Geometry check sheet. Reference: the model listing, model coordinates, mm. A direction names the side the tool comes from. Coordinates: 2 decimals unless noted, no trailing zeros. Order: outer loops, then holes, each group sorted by start corner. A loop starts at its lowest first (then second) coordinate and runs counter-clockwise, first axis right, second up. Notation, with made-up numbers: (37, -9) - (78, -9) arc R23 cw to (78, 19) - close; hole circle Ø5 at (21, 79.25). An arc over 180 degrees is marked (long way). Return JSON: item names as keys, results as strings. Group by question number.
Item 1: Section check C-C on z = -64.5. Enter the section's corners in (x, y).
Item 2: Tool access check on faces 5 (the cylindrical face through (9.99, 1.48, -6.51)), 6 (the flat face through (126.696, 1.479, -57.508)), 7 (the cylindrical face through (120.22, -13.18, -53.68)). Record the directions out of +Z, -Z, +X, -X, +Y, -Y that give a thin tool (end or side, any length) a straight path to the whole face; none if there is none.
Item 3: Gauge pin test, flat ends, axial feed: pin 1 (10 mm diameter, centred on x = 111.5, y = -14.5, fed in from -Z); pin 2 (7 mm diameter, centred on x = 78.3, z = -103.09, fed in from -Y); pin 3 (1.5 mm diameter, centred on x = 43.5, y = 1.5, fed in from -Z); pin 4 (8 mm diameter, centred on y = -11, z = -32.5, fed in from -X). Record the tip position at first contact, or that the pin passes through.
Item 4: Section check B-B on x = 57.5. Enter the section's corners in (y, z) (3 decimals), then the cut area to 3 significant figures.
Item 5: Scan lines: probe 1 along Y at (x, z) = (29.5, -41); probe 2 along Z at (x, y) = (75.5, -16); probe 3 along X at (y, z) = (-24.25, -40.5). Record each from-to range of solid material in increasing order.
Item 6: Draft check along Z on faces 1 (the cylindrical face through (78.43, 1.48, -113.09)), 2 (the flat face through (123, -26, -55)), 3 (the cylindrical face through (-10.68, 1.48, 3.21)), 4 (the flat face through (41.653, 1.479, -20.825)). Enter one of: pulls with the +Z half, pulls with the -Z half, needs draft (parallel to the pull), parting line crosses it, or undercut.
Item 7: Section check A-A on y = -11. Enter the section's corners in (x, z) (3 decimals), then the cut area to 3 significant figures.
Item 8: Section check D-D on z = -13. Enter the section's corners in (x, y).
from build123d import *

# Parameters (mm, degrees)
SKETCH1_R           = 3
SKETCH1_R_2         = 2
BOSS_EXTRUDE1_DEPTH = 3
BOSS_EXTRUDE2_START = -26
SKETCH1_4_R         = 4
SKETCH1_4_R_2       = 2
BOSS_EXTRUDE2_DEPTH = 26


with BuildPart() as part:
    # Sketch1 → Boss-Extrude1 (new body)
    with BuildSketch(Plane(origin=(0, 0, 0), x_dir=(1, 0, 0), z_dir=(0, 1, 0))):
        with BuildLine():
            ThreePointArc((158.22466969, -8.975009298), (167.21501885, -3.353778756), (166.098002955, 7.190266308))
            Line((166.098002955, 7.190266308), (86.175088728, 109.255409789))
            ThreePointArc((86.175088728, 109.255409789), (78.301755463, 113.090134184), (70.428422197, 109.255409789))
            Line((70.428422197, 109.255409789), (-9.49449203, 7.190266308))
            ThreePointArc((-9.49449203, 7.190266308), (-10.611507924, -3.353778756), (-1.621158764, -8.975009298))
            Line((-1.621158764, -8.975009298), (78.301755463, -8.975009298))
            Line((78.301755463, -8.975009298), (158.22466969, -8.975009298))
        make_face()
        with Locations(Location((0, 0, 0), (0, 0, 270))):
            Circle(SKETCH1_R, mode=Mode.SUBTRACT)
        with BuildLine():
            ThreePointArc((18.910520844, 1.024990702), (9.920171683, 6.646221244), (11.037187578, 17.190266308))
            Line((11.037187578, 17.190266308), (28.959351543, 40.077672933))
            Line((28.959351543, 40.077672933), (54.70682481, 1.024990702))
            Line((54.70682481, 1.024990702), (18.910520844, 1.024990702))
        make_face(mode=Mode.SUBTRACT)
        Polygon((59.887035288, 79.573711202), (66.6846286, 79.573711202), (66.6846286, 19.192418643), (41.964871323, 56.686304577), align=None, mode=Mode.SUBTRACT)
        with Locations(Location((78.301755463, -3.975009298, 0), (0, 0, 270))):
            Circle(SKETCH1_R_2, mode=Mode.SUBTRACT)
        with BuildLine():
            Line((156.244075902, -3), (148.244075902, -3))
            ThreePointArc((148.244075902, -3), (145.244075902, 0), (148.244075902, 3))
            Line((148.244075902, 3), (156.244075902, 3))
            ThreePointArc((156.244075902, 3), (159.244075902, 0), (156.244075902, -3))
        make_face(mode=Mode.SUBTRACT)
        with BuildLine():
            Line((137.692990082, 1.024990702), (101.896686116, 1.024990702))
            Line((101.896686116, 1.024990702), (127.644159383, 40.077672933))
            Line((127.644159383, 40.077672933), (145.566323348, 17.190266308))
            ThreePointArc((145.566323348, 17.190266308), (146.683339242, 6.646221244), (137.692990082, 1.024990702))
        make_face(mode=Mode.SUBTRACT)
        with Locations(Location((78.301755463, 40.077672933, 0), (0, 0, 270))):
            Circle(SKETCH1_R_2, mode=Mode.SUBTRACT)
        Polygon((114.638639603, 56.686304577), (89.918882326, 19.192418643), (89.918882326, 79.573711202), (96.716475638, 79.573711202), align=None, mode=Mode.SUBTRACT)
        with Locations(Location((32.47996742, 52.815460811, 0), (0, 0, 270))):
            Circle(SKETCH1_R_2, mode=Mode.SUBTRACT)
        with Locations(Location((78.301755463, 103.090134184, 0), (0, 0, 270))):
            Circle(SKETCH1_R, mode=Mode.SUBTRACT)
        with Locations(Location((124.123543506, 52.815460811, 0), (0, 0, 270))):
            Circle(SKETCH1_R_2, mode=Mode.SUBTRACT)
    extrude(amount=BOSS_EXTRUDE1_DEPTH)

    # Sketch1_4 → Boss-Extrude2 (add)
    # profile 1 of 4: a face of its own
    with BuildSketch(Plane(origin=(0, 0, 0), x_dir=(1, 0, 0), z_dir=(0, 1, 0)).offset(BOSS_EXTRUDE2_START)):
        with Locations(Location((32.47996742, 52.815460811, 0), (0, 0, 270))):
            Circle(SKETCH1_4_R)
        with Locations(Location((32.47996742, 52.815460811, 0), (0, 0, 270))):
            Circle(SKETCH1_4_R_2, mode=Mode.SUBTRACT)
    # profile 2 of 4: a face of its own
    with BuildSketch(Plane(origin=(0, 0, 0), x_dir=(1, 0, 0), z_dir=(0, 1, 0)).offset(BOSS_EXTRUDE2_START)):
        with Locations(Location((124.123543506, 52.815460811, 0), (0, 0, 270))):
            Circle(SKETCH1_4_R)
        with Locations(Location((124.123543506, 52.815460811, 0), (0, 0, 90))):
            Circle(SKETCH1_4_R_2, mode=Mode.SUBTRACT)
    # profile 3 of 4: a face of its own
    with BuildSketch(Plane(origin=(0, 0, 0), x_dir=(1, 0, 0), z_dir=(0, 1, 0)).offset(BOSS_EXTRUDE2_START)):
        with Locations(Location((78.301755463, 40.077672933, 0), (0, 0, 270))):
            Circle(SKETCH1_4_R)
        with Locations(Location((78.301755463, 40.077672933, 0), (0, 0, 270))):
            Circle(SKETCH1_4_R_2, mode=Mode.SUBTRACT)
    # profile 4 of 4: a face of its own
    with BuildSketch(Plane(origin=(0, 0, 0), x_dir=(1, 0, 0), z_dir=(0, 1, 0)).offset(BOSS_EXTRUDE2_START)):
        with Locations(Location((78.301755463, -3.975009298, 0), (0, 0, 270))):
            Circle(SKETCH1_4_R)
        with Locations(Location((78.301755463, -3.975009298, 0), (0, 0, 270))):
            Circle(SKETCH1_4_R_2, mode=Mode.SUBTRACT)
    extrude(amount=BOSS_EXTRUDE2_DEPTH)


solid = part.part
Computed:
{
 "1": {"outline": "(35.38, 0) - (48.08, 0) - (48.08, 3) - (35.38, 3) - close; (66.68, 0) - (89.92, 0) - (89.92, 3) - (66.68, 3) - close; (108.52, 0) - (121.22, 0) - (121.22, 3) - (108.52, 3) - close"},
 "2": {"face 5": "+Y, -Y", "face 6": "-Z, +X, +Y, -Y", "face 7": "-Y"},
 "3": {"pin 1": "passes through", "pin 2": "stops at y = 0", "pin 3": "stops at z = -75.82", "pin 4": "stops at x = 76.51"},
 "4": {"outline": "(0, -92.745) - (3, -92.745) - (3, -76.525) - (0, -76.525) - close; (0, -33.123) - (3, -33.123) - (3, 8.975) - (0, 8.975) - close", "area": "175 mm²"},
 "5": {"probe 1": "y = 0 to 3", "probe 2": "z = -42.93 to -37.22, 1.12 to 6.83", "probe 3": "x = 74.32 to 76.35, 80.26 to 82.28"},
 "6": {"face 1": "pulls with the -Z half", "face 2": "needs draft", "face 3": "parting line crosses it", "face 4": "undercut"},
 "7": {"outline": "circle Ø8 at (32.48, -52.815); circle Ø8 at (78.302, -40.078); circle Ø8 at (78.302, 3.975); circle Ø8 at (124.124, -52.815); hole circle Ø4 at (32.48, -52.815); hole circle Ø4 at (78.302, -40.078); hole circle Ø4 at (78.302, 3.975); hole circle Ø4 at (124.124, -52.815)", "area": "151 mm²"},
 "8": {"outline": "(-4.95, 0) - (9.11, 0) - (9.11, 3) - (-4.95, 3) - close; (46.81, 0) - (109.79, 0) - (109.79, 3) - (46.81, 3) - close; (147.5, 0) - (161.55, 0) - (161.55, 3) - (147.5, 3) - close"}
}
